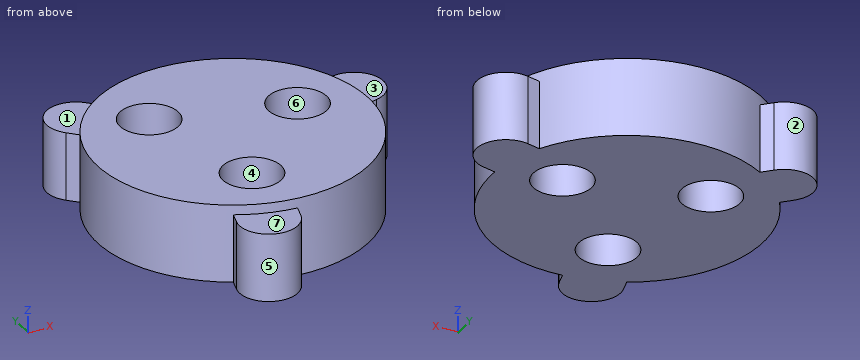
Autodesk Inventor part; units mm, degrees
ref_plane "YZ Plane" through (0, 0, 0) normal (1, 0, 0) x (0, 1, 0)
ref_plane "XZ Plane" through (0, 0, 0) normal (0, 1, 0) x (-1, 0, 0)
ref_plane "XY Plane" through (0, 0, 0) normal (0, 0, 1) x (1, 0, 0)
sketch "スケッチ1" plane through (0, 0, 0) normal (0, 0, 1) x (1, 0, 0)
  circle A0 centre (0, 0) radius 6.975
  circle A1 centre (-2.8284, 2.8284) radius 1.5
  circle A2 centre (-1.0353, -3.8637) radius 1.5
  circle A3 centre (3.8637, 1.0353) radius 1.5
  circle A4 centre (0, 0) radius 9
  line L0 (0, 0) -> (7.2444, 1.9411) construction
  line L1 (0.3882, -1.4489) -> (7.6327, 0.4923)
  line L2 (6.8562, 3.39) -> (-0.3882, 1.4489)
  arc A5 (-0.3882, 1.4489) -> (0.3882, -1.4489) centre (0, 0) ccw
  arc A6 (7.6327, 0.4923) -> (6.8562, 3.39) centre (7.2444, 1.9411) ccw
  arc A7 (-4.2426, 6.364) -> (-6.364, 4.2426) centre (-5.3033, 5.3033) ccw
  line L3 (1.0607, 1.0607) -> (-4.2426, 6.364)
  line L4 (-6.364, 4.2426) -> (-1.0607, -1.0607)
  arc A8 (-3.39, -6.8562) -> (-0.4923, -7.6327) centre (-1.9411, -7.2444) ccw
  line L5 (-1.4489, 0.3882) -> (-3.39, -6.8562)
  line L6 (-0.4923, -7.6327) -> (1.4489, -0.3882)
  point P0 (3.6222, 0.9706)
  point P1 (6.1915, 3.2119)
  point P2 (6.9679, 0.3141)
  point P3 (-5.8773, 3.756)
  point P4 (-3.756, 5.8773)
  point P5 (-0.3141, -6.9679)
  point P6 (-3.2119, -6.1915)
  dimension "d0" = 13.95
  dimension "d1" = 3
  dimension "d2" = 4
  dimension "d5" = 360
  dimension "d9" = 18
  dimension "d14" = 3
  dimension "d17" = 360
extrude "押し出し2" add sketch "スケッチ1" along normal blind 4 contours A0 L6 L1 | L1 A3 L2 A0 | A0 L5 A2 L6 | L2 L3 A0 | L1 A5 L2 A3 | A0 L4 L5 | A2 L5 L4 A5 L1 L6 | L3 A1 L4 A0 | L3 L2 A5 L5 L4 A1 | L5 A5 L4
extrude "押し出し3" add sketch "スケッチ1" along normal blind 3.5 contours A0 L2 A6 L1 | L6 A8 L5 A0 | A0 L4 A7 L3
properties part number "アームカムFD18t4" material "アセタール樹脂、白"
CAD build for the part. Positions are in the model's coordinates, mm. Face numbers are marked on the shaded views. A direction names the side the tool comes from. Round coordinates to 2 decimals unless told otherwise and drop trailing zeros. Loops run counter-clockwise (first coordinate to the right, second up) from the corner with the lowest first, then second, coordinate; pieces in that order, holes last. Notation, with made-up numbers: M -4.5,-36.5 L 7.5,-36.5 A18 ccw 7.5,-27.5 Z; hole C 31,83 d7. An arc over 180 degrees is marked long. Return JSON: item names as keys, results as strings. Group by question number.
(1) Saw through at A-A, the plane y = 0. List the corners of the cut face in (x, z) (3 decimals).
(2) Saw through at B-B, the plane x = -1.75. List the corners of the cut face in (y, z).
(3) Drop flat-ended pins along their axis: P1, Ø3, axis at x = -1, y = -7.5, coming from the +Z side; P2, Ø0.9, axis at x = -5.5, y = 6, coming from the +Z side. Give the stop position or say it passes through.
(4) Mould opens along X. For the marked faces 4, 5, 6 and 7 say: +X half, -X half, draft (parallel to the pull), parting line (faces both ways), or undercut.
(5) Saw through at C-C, the plane y = 2.25. List the corners of the cut face in (x, z), and give its area (3 significant figures).
(6) Wall check: probe 1 along Y at (x, z) = (-2.25, 2.6); probe 2 along Y at (x, z) = (-1, 2.6); probe 3 along Y at (x, z) = (3.75, 1.45). Give the ranges that are in metal, low to high. Write a range as [from, to].
(7) Tool access for the marked faces 1, 2 and 3: list every direction of +Z, -Z, +X, -X, +Y, -Y with a clear straight run to the whole face (end or side of a thin tool).
(8) Saw through at D-D, the plane x = 0. List the corners of the cut face in (y, z) (3 decimals).
Answer list:
{
 "1": {"outline": "M -6.975,0 L 2.778,0 L 2.778,4 L -6.975,4 Z; M 4.949,0 L 6.975,0 L 6.975,4 L 4.949,4 Z"},
 "2": {"outline": "M -8.73,0 L -5.18,0 L -5.18,4 L -6.75,4 L -6.75,3.5 L -8.73,3.5 Z; M -2.54,0 L 1.79,0 L 1.79,4 L -2.54,4 Z; M 3.87,0 L 6.75,0 L 6.75,4 L 3.87,4 Z"},
 "3": {"P1": "z = 4", "P2": "z = 3.5"},
 "4": {"face 4": "undercut", "face 5": "parting line", "face 6": "undercut", "face 7": "draft"},
 "5": {"outline": "M -6.6,0 L -4.21,0 L -4.21,4 L -6.6,4 Z; M -1.44,0 L 2.98,0 L 2.98,4 L -1.44,4 Z; M 4.74,0 L 8.71,0 L 8.71,3.5 L 6.6,3.5 L 6.6,4 L 4.74,4 Z", "area": "42.1 mm2"},
 "6": {"probe 1": "[-8.71, -4.74], [-2.98, 1.44], [4.21, 6.6]", "probe 2": "[-8.41, -5.36], [-2.36, 6.9]", "probe 3": "[-5.88, -0.46], [2.53, 5.88]"},
 "7": {"face 1": "+Z, -X, +Y", "face 2": "+Z, -Z", "face 3": "+Z, +X, +Y"},
 "8": {"outline": "M -6.975,0 L -4.949,0 L -4.949,4 L -6.975,4 Z; M -2.778,0 L 6.975,0 L 6.975,4 L -2.778,4 Z"}
}
